```python
from build123d import *

# Parameters (mm, degrees)
F2_R     = 2.75
F3_DEPTH = 25
F5_D     = 4.2
F5_DEPTH = 22.4
F5_TIP   = 1.2618073


with BuildPart() as f1:
    # F0 (on Front) → F1 (revolve)
    with BuildSketch(Plane.XZ):
        with BuildLine():
            Line((-166.1916986587, 0), (-163.1916986587, 0))
            Line((-163.1916986587, 0), (136.8083013413, 0))
            Line((136.8083013413, 0), (136.8083013413, 20))
            Line((136.8083013413, 20), (-97.1916986587, 20))
            Line((-97.1916986587, 20), (-107.1916986587, 10))
            Line((-107.1916986587, 10), (-156.6916986587, 10))
            ThreePointArc((-156.6916986587, 10), (-157.0452520493, 10.1464466094), (-157.1916986587, 10.5))
            Line((-157.1916986587, 10.5), (-157.1916986587, 20))
            Line((-157.1916986587, 20), (-163.1916986587, 20))
            Line((-163.1916986587, 20), (-163.1916986587, 10.5))
            ThreePointArc((-163.1916986587, 10.5), (-163.3381452681, 10.1464466094), (-163.6916986587, 10))
            Line((-163.6916986587, 10), (-166.1916986587, 10))
            Line((-166.1916986587, 10), (-166.1916986587, 0))
        make_face()
    revolve(axis=Axis((-0.7568523288, 0, 0), (1, 0, 0)))

    # F2 (on face) → F3 (cut)
    with BuildSketch(Plane(origin=(-163.1916986587, 0, 0), x_dir=(0, -1, 0), z_dir=(-1, 0, 0))):
        with Locations((0, 15.75)):
            Circle(F2_R)
        with Locations((-11.1369318037, 11.1369318037)):
            Circle(F2_R)
        with Locations((-11.1369318037, -11.1369318037)):
            Circle(F2_R)
        with Locations((11.1369318037, -11.1369318037)):
            Circle(F2_R)
        with Locations((11.1369318037, 11.1369318037)):
            Circle(F2_R)
    extrude(amount=-F3_DEPTH, mode=Mode.SUBTRACT)

    # F5
    with Locations(Plane.YZ.offset(136.8083013413)):
        with Locations((0, 15), (0, -15)):
            Hole(F5_D / 2, depth=F5_DEPTH)
            with Locations((0, 0, -(F5_DEPTH + F5_TIP / 2))):  # 118° drill point
                Cone(0, F5_D / 2, F5_TIP, mode=Mode.SUBTRACT)


solid = f1.part
```
Check sheet for the modelled part. Datum: model origin and axes. Units: mm. A direction names the side the tool comes from. Round coordinates to 2 decimals unless told otherwise and drop trailing zeros. Order: outer loops, then holes, each group sorted by start corner. A loop starts at its lowest first (then second) coordinate and runs counter-clockwise, first axis right, second up. Notation, with made-up numbers: (81, 19.25) -> (135, 19.25) arc R33 ccw to (135, 51.25) -> close; hole circle Ø4 at (-22.5, -36). An arc over 180 degrees is marked (long way). One line per item, written item: value. Start each with the question number.
Q1. Mould release check, pull along X, two halves, no side actions. Record for faces 4 (the face through (136.808, 0, 0)), 5 (the face through (-132.29, 9.76, -2.17)), 6 (the face through (-166.192, 0, 0)), 7 (the face through (-164.96, 9.76, -2.17)): pulls with the +X half, pulls with the -X half, needs draft (parallel to the pull), parting line crosses it, or undercut.
Q2. Set-up check for faces 1 (the face through (-160.234, 0.358, 18.477)), 2 (the face through (-160.234, 19.524, -4.336)), 3 (the face through (-157.192, 9, -9)): record each of +Z, -Z, +X, -X, +Y, -Y from which the full face is reachable in a straight line by a thin tool's end or side.
Q3. Cross-section at C-C (x = -145.5). Record the boundary of the cut face in (y, z).
Q4. Cross-section at A-A (z = 0). Record the boundary of the cut face in (x, y), and give its area (3 significant figures).
Q5. Gauge pin test, flat ends, axial feed: pin 1 Ø8 at (x, z) = (-38.5, -6) entering from +Y; pin 2 Ø1.5 at (x, y) = (-130.5, -3) entering from +Z; pin 3 Ø4 at (y, z) = (0, 15) entering from +X. Record the tip position at first contact, or that the pin passes through.
Q6. Cross-section at B-B (x = -17). Record the boundary of the cut face in (y, z), and give its area (3 significant figures).
Q7. Thickness scan on line 1 (Z direction, x = -161, y = 0); line 2 (Z direction, x = 123.5, y = 1.5); line 3 (X direction, y = -16, z = 4). Record the ranges inside material, lowest first.
Completed:
1. face 4: pulls with the +X half
1. face 5: undercut
1. face 6: pulls with the -X half
1. face 7: needs draft
2. face 1: -X
2. face 2: +X, -X
2. face 3: none
3. outline: circle Ø20 at (0, 0)
4. outline: (-166.19, -10) -> (-163.69, -10) arc R0.5 cw to (-163.19, -10.5) -> (-163.19, -20) -> (-157.19, -20) -> (-157.19, -10.5) arc R0.5 cw to (-156.69, -10) -> (-107.19, -10) -> (-97.19, -20) -> (136.81, -20) -> (136.81, 20) -> (-97.19, 20) -> (-107.19, 10) -> (-156.69, 10) arc R0.5 cw to (-157.19, 10.5) -> (-157.19, 20) -> (-163.19, 20) -> (-163.19, 10.5) arc R0.5 cw to (-163.69, 10) -> (-166.19, 10) -> close
4. area: 11,000 mm²
5. pin 1: stops at y = 19.9
5. pin 2: stops at z = 9.74
5. pin 3: stops at x = 114.35
6. outline: circle Ø40 at (0, 0)
6. area: 1,260 mm²
7. line 1: z = -20 to 13, 18.5 to 20
7. line 2: z = -19.94 to -16.47, -13.53 to 13.53, 16.47 to 19.94
7. line 3: x = -163.19 to -157.19, -100.7 to 136.81
